Verification items for the finished model (mm, model axes). Coordinates: 2 decimals unless noted, no trailing zeros. Order: outer loops, then holes, each group sorted by start corner. A loop starts at its lowest first (then second) coordinate and runs counter-clockwise, first axis right, second up. Notation, with made-up numbers: (6.5, 52.25) -> (59.5, 52.25) arc R15 ccw to (59.5, 78.25) -> close; hole circle Ø9 at (36.25, 35). An arc over 180 degrees is marked (long way). Write item = value, one per line. Start each with the question number.
1. Thickness scan on line 1 along Z through (x, y) = (0, 1.8); line 2 along Z through (x, y) = (75, 3.75); line 3 along X through (y, z) = (1.7, -3.25). Record the ranges inside material, lowest first. Write a range as from..to.
2. Go/stop test with a flat-tipped pin: P1, Ø2, axis at y = 3, z = -3, coming from the +X side. Record where the tip stops, or that it passes through.
3. Cross-section at A-A on x = 0. Record the cut outline in (y, z), plus the area to 3 significant figures.
4. Release check for a two-part mould opening along Z. For faces 1 (the flat face through (-1, 2, -12.5)), 2 (the cylindrical face through (-1.08, 2.46, -4.88)), 3 (the cylindrical face through (71, 2, 0)), 4 (the flat face through (1, 0, 6)) record: +Z half, -Z half, draft (parallel to the pull), parting line (faces both ways), or undercut.
5. Cross-section at C-C on y = 1.15. Record the cut outline in (x, z).
6. Cross-section at D-D on z = -10.5. Record the cut outline in (x, y), plus the area to 3 significant figures.
7. Cross-section at B-B on z = 0. Record the cut outline in (x, y).
Solid Edge part; units mm, degrees
sketch "Sketch1" plane through (0, 0, 0) normal (0, -1, 0) x (1, 0, 0)
  line L0 (75, 12.5) -> (-75, 12.5)
  line L1 (-75, -12.5) -> (75, -12.5)
  arc A0 (-75, -12.5) -> (-75, 12.5) centre (-75, 0) cw
  arc A1 (75, 12.5) -> (75, -12.5) centre (75, 0) cw
  circle A2 centre (-75, 0) radius 3
  circle A3 centre (75, 0) radius 4
  circle A4 centre (0, 0) radius 5
extrude "ExtrudedProtrusion_2" add sketch "Sketch1" against normal blind 5
properties material "Polycarbonate( 20-40% Glass Fiber)"
Worked out:
q1.line_1 = -12.5..-5, 5..12.5
q1.line_2 = -12.5..-4, 4..12.5
q1.line_3 = -87.07..-3.8, 3.8..72.67, 77.33..87.07
q2.P1 = 87.34
q3.outline = (0, -12.5) -> (5, -12.5) -> (5, -5) -> (0, -5) -> close; (0, 5) -> (5, 5) -> (5, 12.5) -> (0, 12.5) -> close
q3.area = 75.0 mm²
q4.face_1 = -Z half
q4.face_2 = undercut
q4.face_3 = undercut
q4.face_4 = draft
q5.outline = (-75, -12.5) -> (75, -12.5) arc R12.5 ccw to (75, 12.5) -> (-75, 12.5) arc R12.5 ccw to start; hole circle Ø6 at (-75, 0); hole circle Ø10 at (0, 0); hole circle Ø8 at (75, 0)
q6.outline = (-81.78, 0) -> (81.78, 0) -> (81.78, 5) -> (-81.78, 5) -> close
q6.area = 818 mm²
q7.outline = (-87.5, 0) -> (-78, 0) -> (-78, 5) -> (-87.5, 5) -> close; (-72, 0) -> (-5, 0) -> (-5, 5) -> (-72, 5) -> close; (5, 0) -> (71, 0) -> (71, 5) -> (5, 5) -> close; (79, 0) -> (87.5, 0) -> (87.5, 5) -> (79, 5) -> close
